Work out the finished part from the listing and answer in its coordinate system (mm). Face numbers are marked on the shaded views. A direction names the side the tool comes from. Coordinates: 2 decimals unless noted, no trailing zeros. Loops run counter-clockwise (first coordinate to the right, second up) from the corner with the lowest first, then second, coordinate; pieces in that order, holes last. Notation, with made-up numbers: M 52,35.5 L 82,35.5 A14 cw 82,51.5 Z; hole C -7,-19 d10. An arc over 180 degrees is marked long. Write each question's results on one line, items separated by ' | '.
```python
from build123d import *

# Parameters (mm, degrees)
SKETCH1_W               = 19.05
SKETCH1_H               = 19.05
BOSS_EXTRUDE1_DEPTH     = 8
SKETCH2_R               = 2.75
CUT_EXTRUDE1_DEPTH      = 6
CUT_EXTRUDE2_DEPTH      = 29.103469537
CUT_EXTRUDE2_DEPTH_BACK = 29.103469537
SKETCH2_3_R             = 2.75
FILLET1_R               = 1.5


with BuildPart() as part:
    # Sketch1 → Boss-Extrude1 (new body)
    with BuildSketch(Plane.XY):
        with Locations((9.525, 9.525)):
            Rectangle(SKETCH1_W, SKETCH1_H)
    extrude(amount=BOSS_EXTRUDE1_DEPTH)

    # Sketch2 → Cut-Extrude1 (cut)
    # profile 1 of 2: a face of its own
    with BuildSketch(Plane.XY.offset(8)):
        Polygon((7.143430137, 5.399999995), (11.906569863, 5.399999995), (14.288139727, 9.525), (11.906569863, 13.650000005), (7.143430137, 13.650000005), (4.761860273, 9.525), align=None)
        with Locations((9.525, 9.525)):
            Circle(SKETCH2_R, mode=Mode.SUBTRACT)
    # profile 2 of 2: a face of its own
    with BuildSketch(Plane.XY.offset(8)):
        with Locations((9.525, 9.525)):
            Circle(SKETCH2_R)
    extrude(amount=-CUT_EXTRUDE1_DEPTH, mode=Mode.SUBTRACT)

    # Sketch2<3> → Cut-Extrude2 (cut, two sides: drawn at the far end of the back side and taken through both)
    with BuildSketch(Plane.XY.offset(8).offset(-CUT_EXTRUDE2_DEPTH_BACK)):
        with Locations((9.525, 9.525)):
            Circle(SKETCH2_3_R)
    extrude(amount=CUT_EXTRUDE2_DEPTH + CUT_EXTRUDE2_DEPTH_BACK, mode=Mode.SUBTRACT)

    # Fillet1
    fillet1_edges = [part.edges().sort_by_distance(p)[0] for p in [
        (0, 19.05, 4),
        (19.05, 19.05, 4),
        (19.05, 0, 4),
        (0, 0, 4),
    ]]
    fillet(fillet1_edges, radius=FILLET1_R)


solid = part.part
```
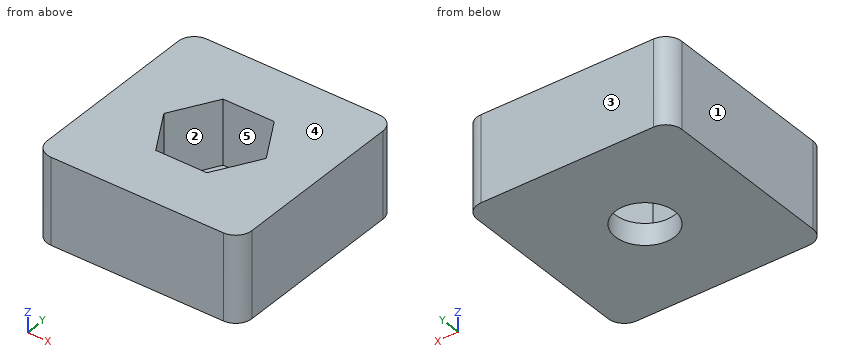
1) For a pull along Y with two mould halves and no side action, classify the marked faces 1, 2 and 3 as released by +Y, released by -Y, zero draft, split by the parting line, or undercut.
Check result:
face 1: zero draft | face 2: undercut | face 3: released by +Y
2) Find section C-C, the plane y = 9. Give the vertices of the cut face in (x, z), and give its area (3 significant figures).
Check result:
outline: M 0,0 L 6.83,0 L 6.83,2 L 5.06,2 L 5.06,8 L 0,8 Z; M 12.22,0 L 19.05,0 L 19.05,8 L 13.99,8 L 13.99,2 L 12.22,2 Z | area: 88.1 mm^2
3) Straight lines are drawn through the part: probe 1 along Y at (x, z) = (8, 3); probe 2 along X at (y, z) = (11.75, 0.5); probe 3 along Y at (x, z) = (7.25, 1). For each, find the intervals that lie inside material, in ascending order. Write a range as [from, to].
Check result:
probe 1: [0, 5.4], [13.65, 19.05] | probe 2: [0, 7.91], [11.14, 19.05] | probe 3: [0, 7.98], [11.07, 19.05]
4) Find section D-D, the plane y = 12.5. Give the vertices of the cut face in (x, z), and give its area (3 significant figures).
Check result:
outline: M 0,0 L 19.05,0 L 19.05,8 L 12.57,8 L 12.57,2 L 6.48,2 L 6.48,8 L 0,8 Z | area: 116 mm^2
5) Which of the six approach directions +Z, -Z, +X, -X, +Y, -Y give full straight-line access (tool end or side, diameter ignored) to the marked faces 4 and 5?
Check result:
face 4: +Z, +X, -X, +Y, -Y | face 5: +Z
6) Find section A-A, the plane z = 1. Give the vertices of the cut face in (x, y) (3 decimals), and give its area (3 significant figures).
Check result:
outline: M 0,1.5 A1.5 ccw 1.5,0 L 17.55,0 A1.5 ccw 19.05,1.5 L 19.05,17.55 A1.5 ccw 17.55,19.05 L 1.5,19.05 A1.5 ccw 0,17.55 Z; hole C 9.525,9.525 d5.5 | area: 337 mm^2
7) Find section B-B, the plane x = 11. Give the vertices of the cut face in (y, z).
Check result:
outline: M 0,0 L 7.2,0 L 7.2,2 L 5.4,2 L 5.4,8 L 0,8 Z; M 11.85,0 L 19.05,0 L 19.05,8 L 13.65,8 L 13.65,2 L 11.85,2 Z
8) Given pin 1 Ø1.5 at (x, y) = (16, 14) entering from -Z; pin 2 Ø4 at (x, y) = (7.5, 9) entering from +Z, each flat-ended and moving along its own axis, determine where each tip first touches the part or whether it passes through.
Check result:
pin 1: z = 0 | pin 2: z = 2
